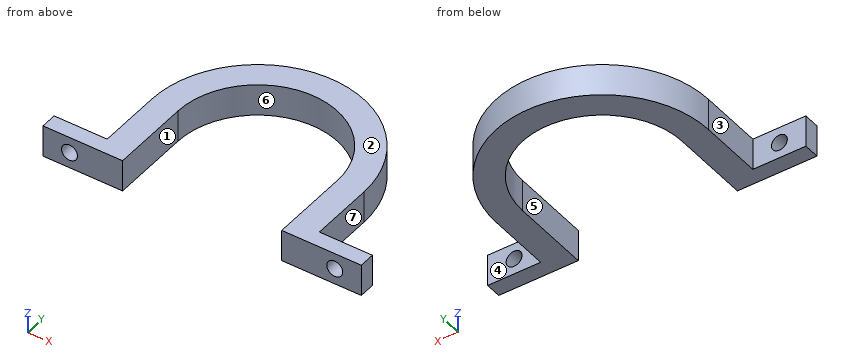
from build123d import *

# Parameters (mm, degrees)
BOSS_EXTRUDE1_DEPTH = 6
SKETCH2_R           = 1.5
CUT_EXTRUDE1_DEPTH  = 3


with BuildPart() as part:
    # Sketch1 → Boss-Extrude1 (new body)
    with BuildSketch(Plane.XY):
        with BuildLine():
            Line((15, 0), (15, -15))
            Line((15, -15), (30, -15))
            Line((30, -15), (30, -12))
            Line((30, -12), (20, -12))
            Line((20, -12), (20, 0))
            ThreePointArc((20, 0), (0, 20), (-20, 0))
            Line((-20, 0), (-20, -12))
            Line((-20, -12), (-30, -12))
            Line((-30, -12), (-30, -15))
            Line((-30, -15), (-15, -15))
            Line((-15, -15), (-15, 0))
            ThreePointArc((-15, 0), (0, 15), (15, 0))
        make_face()
    extrude(amount=BOSS_EXTRUDE1_DEPTH)

    # Sketch2 → Cut-Extrude1 (cut)
    with BuildSketch(Plane(origin=(0, -12, 0), x_dir=(1, 0, 0), z_dir=(0, 1, 0))):
        with Locations((-25, -3)):
            Circle(SKETCH2_R)
        with Locations((25, -3)):
            Circle(SKETCH2_R)
    extrude(amount=-CUT_EXTRUDE1_DEPTH, mode=Mode.SUBTRACT)


solid = part.part
The model under review builds one solid part; all positions refer to its coordinate system, in mm. Face numbers are marked on the shaded views. A direction names the side the tool comes from. Give positions to 0.01 mm unless a question says otherwise; leave off trailing zeros. Loops run counter-clockwise (first coordinate to the right, second up) from the corner with the lowest first, then second, coordinate; pieces in that order, holes last. Notation, with made-up numbers: (41, 42.5) -> (51, 42.5) arc R26 ccw to (51, 78.5) -> close; hole circle Ø9 at (26.25, -2). An arc over 180 degrees is marked (long way). Write each question's results on one line, items separated by ' | '.
1) Insertion check: pin 1 Ø1.8 at (y, z) = (-11, 1.5) entering from +X; pin 2 Ø1.8 at (x, z) = (25, 3) entering from +Y; pin 3 Ø3 at (y, z) = (6, 1) entering from +X; pin 4 Ø1 at (y, z) = (1, 3) entering from -X. Each pin has a flat end and moves straight along its axis. Give the tip position at first contact, or say it passes through.
Conclusion:
pin 1: stops at x = 20 | pin 2: passes through | pin 3: stops at x = 19.49 | pin 4: stops at x = -19.99
2) Take a section at A-A, the plane x = -25. Give the boundary of the cut face in (y, z), plus the area to 3 significant figures.
Conclusion:
outline: (-15, 0) -> (-12, 0) -> (-12, 1.5) -> (-15, 1.5) -> close; (-15, 4.5) -> (-12, 4.5) -> (-12, 6) -> (-15, 6) -> close | area: 9.00 mm^2
3) Tool access review of the marked faces 1, 2 and 3: name each direction out of +Z, -Z, +X, -X, +Y, -Y from which nothing blocks a thin tool from reaching the whole face with its end or side.
Conclusion:
face 1: +Z, -Z, -Y | face 2: +Z, +X, -X, +Y, -Y | face 3: +Z, -Z, -X, +Y
4) Take a section at D-D, the plane x = 0. Give the boundary of the cut face in (y, z).
Conclusion:
outline: (15, 0) -> (20, 0) -> (20, 6) -> (15, 6) -> close
5) Take a section at C-C, the plane y = 9.5. Give the boundary of the cut face in (x, z), plus the area to 3 significant figures.
Conclusion:
outline: (-17.6, 0) -> (-11.61, 0) -> (-11.61, 6) -> (-17.6, 6) -> close; (11.61, 0) -> (17.6, 0) -> (17.6, 6) -> (11.61, 6) -> close | area: 71.9 mm^2
6) For line 1 along X through (y, z) = (-12.85, 3); line 2 along Z through (x, y) = (-25, -14.3); line 3 along X through (y, z) = (-4.5, 5), list the stretches that pass through material, from the lowest coordinate up. Write a range as from..to.
Conclusion:
line 1: x = -30..-26.5, -23.5..-15, 15..23.5, 26.5..30 | line 2: z = 0..1.5, 4.5..6 | line 3: x = -20..-15, 15..20
7) Take a section at B-B, the plane z = 3. Give the boundary of the cut face in (x, y), plus the area to 3 significant figures.
Conclusion:
outline: (-30, -15) -> (-26.5, -15) -> (-26.5, -12) -> (-30, -12) -> close; (-23.5, -15) -> (-15, -15) -> (-15, 0) arc R15 cw to (15, 0) -> (15, -15) -> (23.5, -15) -> (23.5, -12) -> (20, -12) -> (20, 0) arc R20 ccw to (-20, 0) -> (-20, -12) -> (-23.5, -12) -> close; (26.5, -15) -> (30, -15) -> (30, -12) -> (26.5, -12) -> close | area: 467 mm^2
8) Draft analysis for pull direction X (two halves, no side actions). For the marked faces 4, 5, 6 and 7, state which applies: pulls with the +X half, pulls with the -X half, needs draft (parallel to the pull), parting line crosses it, or undercut.
Conclusion:
face 4: needs draft | face 5: undercut | face 6: undercut | face 7: pulls with the +X half
